from build123d import *

# Parameters (mm, degrees)
SKETCH_1_R          = 2
SKETCH_1_R_2        = 4.5
EXTRUDE_1_DEPTH     = 4
SKETCH_2_R          = 1.5
SKETCH_2_W          = 4.4
SKETCH_2_H          = 8.4
CUT_EXTRUDE_1_DEPTH = 4
SKETCH_3_W          = 87
SKETCH_3_H          = 3.5
EXTRUDE_2_DEPTH     = 4


with BuildPart() as part:
    # 草图1 → 凸台-拉伸1 (new body)
    with BuildSketch(Plane.XY):
        Polygon((37.5, 50), (-37.5, 50), (-43.5, 50), (-43.5, -57), (-43.5, -164), (-37.5, -164), (37.5, -164), (43.5, -164), (43.5, -57), (43.5, 50), align=None)
        with Locations((-37.5, -126)):
            Circle(SKETCH_1_R, mode=Mode.SUBTRACT)
        Polygon((-27.5, -128.391668474), (-27.5, -51), (19.690041753, -51), align=None, mode=Mode.SUBTRACT)
        Polygon((-19.690041753, -154), (27.5, -76.608331526), (27.5, -154), align=None, mode=Mode.SUBTRACT)
        with Locations((-37.5, -41)):
            Circle(SKETCH_1_R, mode=Mode.SUBTRACT)
        with Locations((-20, -40)):
            Circle(SKETCH_1_R, mode=Mode.SUBTRACT)
        with Locations((-37.5, 44)):
            Circle(SKETCH_1_R, mode=Mode.SUBTRACT)
        with Locations((-20, 0)):
            Circle(SKETCH_1_R, mode=Mode.SUBTRACT)
        Circle(SKETCH_1_R_2, mode=Mode.SUBTRACT)
        with Locations((-20, 40)):
            Circle(SKETCH_1_R, mode=Mode.SUBTRACT)
        with Locations((20, -40)):
            Circle(SKETCH_1_R, mode=Mode.SUBTRACT)
        with Locations((20, 0)):
            Circle(SKETCH_1_R, mode=Mode.SUBTRACT)
        with Locations((20, 40)):
            Circle(SKETCH_1_R, mode=Mode.SUBTRACT)
        with Locations((37.5, 44)):
            Circle(SKETCH_1_R, mode=Mode.SUBTRACT)
    extrude(amount=EXTRUDE_1_DEPTH)

    # 草图2 → 切除-拉伸1 (cut)
    with BuildSketch(Plane.XY.offset(4)):
        with Locations((37.5, -158)):
            Circle(SKETCH_2_R)
        with Locations((37.5, -78)):
            Circle(SKETCH_2_R)
        with Locations((37.5, -118)):
            Circle(SKETCH_2_R)
        with Locations((37.5, -138)):
            Rectangle(SKETCH_2_W, SKETCH_2_H)
        with Locations((37.5, -98)):
            Rectangle(SKETCH_2_W, SKETCH_2_H)
        with Locations((37.5, -58)):
            Rectangle(SKETCH_2_W, SKETCH_2_H)
    extrude(amount=-CUT_EXTRUDE_1_DEPTH, mode=Mode.SUBTRACT)

    # 草图3 → 凸台-拉伸2 (add)
    with BuildSketch(Plane.XY.offset(4)):
        with Locations((0, -165.75)):
            Rectangle(SKETCH_3_W, SKETCH_3_H)
    extrude(amount=-EXTRUDE_2_DEPTH)


solid = part.part
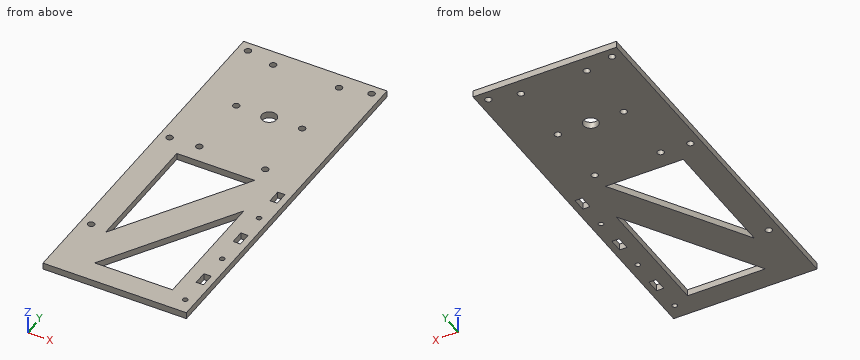
Build history of the part. All positions in model axes, mm. Round coordinates to 2 decimals unless told otherwise and drop trailing zeros. Write each loop counter-clockwise with the first axis right and the second up, starting at its lowest first coordinate (ties: lowest second). Pieces come first, ordered by that corner, then holes. Notation, with made-up numbers: M 3,7 L 49,7 A34 ccw 49,39 Z; hole C -9.75,27.25 d3. An arc over 180 degrees is marked long. Answer in a Markdown table with one row per item.
1. Probe L1, parallel to Y at x = -37.5, z = 1.4; L2, parallel to Y at x = 0, z = 1.4; L3, parallel to Y at x = -8, z = 3.6. List the from-to ranges inside material, lowest first. Write a range as [from, to].
Geometry check:
| item | result |
|---|---|
| L1 | [-167.5, -128], [-124, -43], [-39, 42], [46, 50] |
| L2 | [-167.5, -154], [-121.71, -83.29], [-51, -4.5], [4.5, 50] |
| L3 | [-167.5, -154], [-134.83, -96.41], [-51, 50] |
2. Saw through at A-A (y = 44). List the corners of the cut face in (x, z).
Geometry check:
| item | result |
|---|---|
| outline | M -43.5,0 L -39.5,0 L -39.5,4 L -43.5,4 Z; M -35.5,0 L 35.5,0 L 35.5,4 L -35.5,4 Z; M 39.5,0 L 43.5,0 L 43.5,4 L 39.5,4 Z |
3. Saw through at C-C (x = 7). List the corners of the cut face in (y, z), and give its area (3 significant figures).
Geometry check:
| item | result |
|---|---|
| outline | M -167.5,0 L -154,0 L -154,4 L -167.5,4 Z; M -110.23,0 L -71.81,0 L -71.81,4 L -110.23,4 Z; M -51,0 L 50,0 L 50,4 L -51,4 Z |
| area | 612 mm2 |
4. Saw through at B-B (y = 0). List the corners of the cut face in (x, z).
Geometry check:
| item | result |
|---|---|
| outline | M -43.5,0 L -22,0 L -22,4 L -43.5,4 Z; M -18,0 L -4.5,0 L -4.5,4 L -18,4 Z; M 4.5,0 L 18,0 L 18,4 L 4.5,4 Z; M 22,0 L 43.5,0 L 43.5,4 L 22,4 Z |
5. Saw through at D-D (y = -146). List the corners of the cut face in (x, z), and give its area (3 significant figures).
Geometry check:
| item | result |
|---|---|
| outline | M -43.5,0 L -14.81,0 L -14.81,4 L -43.5,4 Z; M 27.5,0 L 43.5,0 L 43.5,4 L 27.5,4 Z |
| area | 179 mm2 |
